```python
from build123d import *

# Parameters (mm, degrees)
SKETCH1_W           = 50
SKETCH1_H           = 60
SKETCH1_R           = 3
BOSS_EXTRUDE1_DEPTH = 3
SKETCH2_R           = 2
CUT_EXTRUDE1_DEPTH  = 4


with BuildPart() as part:
    # Sketch1 → Boss-Extrude1 (new body)
    with BuildSketch(Plane.XY):
        Rectangle(SKETCH1_W, SKETCH1_H)
        Circle(SKETCH1_R, mode=Mode.SUBTRACT)
    extrude(amount=BOSS_EXTRUDE1_DEPTH)

    # Sketch2 → Cut-Extrude1 (cut, through all)
    with BuildSketch(Plane(origin=(0, 0, 0), x_dir=(-1, 0, 0), z_dir=(0, 0, -1))):
        with Locations((0, 12.5)):
            Circle(SKETCH2_R)
        with Locations((0, -12.5)):
            Circle(SKETCH2_R)
    extrude(amount=-CUT_EXTRUDE1_DEPTH, mode=Mode.SUBTRACT)


solid = part.part
```
Can you work these out from the model? Positions are in its coordinate system, mm. Round coordinates to 2 decimals unless told otherwise and drop trailing zeros. Loops run counter-clockwise (first coordinate to the right, second up) from the corner with the lowest first, then second, coordinate; pieces in that order, holes last. Notation, with made-up numbers: M -12,33.5 L 38,33.5 A12 cw 38,37.5 Z; hole C -17,20.5 d4. An arc over 180 degrees is marked long. Answer in a Markdown table with one row per item.
1. Please list where these lines run through material, in increasing order: line 1 (Y direction, x = 0, z = 2.1); line 2 (Y direction, x = -1.5, z = 0.3). Write a range as from..to.
Established:
| item | result |
|---|---|
| line 1 | -30..-14.5, -10.5..-3, 3..10.5, 14.5..30 |
| line 2 | -30..-13.82, -11.18..-2.6, 2.6..11.18, 13.82..30 |
2. If we section it at B-B, the plane y = 0: Please give me the cut outline in (x, z).
Established:
| item | result |
|---|---|
| outline | M -25,0 L -3,0 L -3,3 L -25,3 Z; M 3,0 L 25,0 L 25,3 L 3,3 Z |
3. If we section it at A-A, the plane x = 0: Please give me the cut outline in (y, z), plus the area to 3 significant figures.
Established:
| item | result |
|---|---|
| outline | M -30,0 L -14.5,0 L -14.5,3 L -30,3 Z; M -10.5,0 L -3,0 L -3,3 L -10.5,3 Z; M 3,0 L 10.5,0 L 10.5,3 L 3,3 Z; M 14.5,0 L 30,0 L 30,3 L 14.5,3 Z |
| area | 138 mm² |
4. Thinking about a two-plate mould opening in X: for faces 1 (the face through (-3, 0, 1)), 2 (the face through (0, 30, 1)), 3 (the face through (0.26, 14.483, 1.479)), 4 (the face through (-25, 0, 1)), which applies, pulls with the +X half, pulls with the -X half, needs draft (parallel to the pull), parting line crosses it, or undercut?
Established:
| item | result |
|---|---|
| face 1 | undercut |
| face 2 | needs draft |
| face 3 | undercut |
| face 4 | pulls with the -X half |
5. If we section it at D-D, the plane y = -12.5: Please give me the cut outline in (x, z).
Established:
| item | result |
|---|---|
| outline | M -25,0 L -2,0 L -2,3 L -25,3 Z; M 2,0 L 25,0 L 25,3 L 2,3 Z |
6. If we section it at C-C, the plane z = 1.1: Please give me the cut outline in (x, y), plus the area to 3 significant figures.
Established:
| item | result |
|---|---|
| outline | M -25,-30 L 25,-30 L 25,30 L -25,30 Z; hole C 0,0 d6; hole C 0,-12.5 d4; hole C 0,12.5 d4 |
| area | 2,950 mm² |
